Build history of the part. All positions in model axes, mm. A direction names the side the tool comes from. Round coordinates to 2 decimals unless told otherwise and drop trailing zeros. Loops run counter-clockwise (first coordinate to the right, second up) from the corner with the lowest first, then second, coordinate; pieces in that order, holes last. Notation, with made-up numbers: (-40, -26.75) -> (-1, -26.75) arc R33 cw to (-1, 1.25) -> close; hole circle Ø7 at (5, 59). An arc over 180 degrees is marked (long way). Put each result on its own line as item: value. Start each with the question number.
Item 1: Cut at D-D, the plane z = 2. List the corners of the cut face in (x, y), plus the area to 3 significant figures.
Item 2: Drill centre lines: probe 1 along Z at (x, y) = (0.5, 2.2); probe 2 along X at (y, z) = (1.9, 4); probe 3 along X at (y, z) = (4.65, 0.25). Where is each one in solid material? Low to high. Write a range as [from, to].
Item 3: Cut at C-C, the plane y = 0.9. List the corners of the cut face in (x, z).
Item 4: Flat gauge pins, fed straight in: pin 1 Ø2 at (x, y) = (1, 2) entering from -Z; pin 2 Ø3 at (x, z) = (0, 4) entering from -Y. Where does each tip first touch, or does it go through?
Item 5: Cut at B-B, the plane z = 5.25. List the corners of the cut face in (x, y), plus the area to 3 significant figures.
Item 6: Cut at A-A, the plane x = 0. List the corners of the cut face in (y, z), plus the area to 3 significant figures.
Item 7: Pull direction X, two halves, no side cores. Call faces 3 (the cylindrical face through (1.05, 0.74, -8.11)), 4 (the flat face through (-7.8, 1.5, -4.4)), 5 (the cylindrical face through (-0.97, 3.04, -5.27)): +X half, -X half, draft (parallel to the pull), parting line (faces both ways), or undercut.
Item 8: Tool access for faces 1 (the cylindrical face through (-1.17, 3.718, -7.493)), 2 (the cylindrical face through (-0.61, 3.04, 5.48)): list every direction of +Z, -Z, +X, -X, +Y, -Y with a clear straight run to the whole face (end or side of a thin tool).
```python
from build123d import *

# Parameters (mm, degrees)
SKETCH1_R           = 7.5
BOSS_EXTRUDE1_DEPTH = 6
SKETCH2_R           = 8.5
BOSS_EXTRUDE2_DEPTH = 1.5
SKETCH4_R           = 1.6
CUT_EXTRUDE1_DEPTH  = 15.43086969


with BuildPart() as part:
    # Sketch1 → Boss-Extrude1 (new body)
    with BuildSketch(Plane(origin=(0, 0, 0), x_dir=(1, 0, 0), z_dir=(0, 1, 0))):
        with Locations(Location((-1.5, 0, 0), (0, 0, 270))):
            Circle(SKETCH1_R)
    extrude(amount=BOSS_EXTRUDE1_DEPTH)

    # Sketch2 → Boss-Extrude2 (add)
    with BuildSketch(Plane.XZ):
        with Locations(Location((-1.5, 0, 0), (0, 0, 270))):
            Circle(SKETCH2_R)
    extrude(amount=-BOSS_EXTRUDE2_DEPTH)

    # Sketch4 → Cut-Extrude1 (cut, through all)
    with BuildSketch(Plane(origin=(0, 6, 0), x_dir=(1, 0, 0), z_dir=(0, 1, 0))):
        with Locations(Location((0, 4, 0), (0, 0, 270))):
            Circle(SKETCH4_R)
        with Locations(Location((0, -4, 0), (0, 0, 270))):
            Circle(SKETCH4_R)
    extrude(amount=-CUT_EXTRUDE1_DEPTH, mode=Mode.SUBTRACT)


solid = part.part
```
Reply:
1. outline: (-9.76, 0) -> (6.76, 0) -> (6.76, 1.5) -> (5.73, 1.5) -> (5.73, 6) -> (-8.73, 6) -> (-8.73, 1.5) -> (-9.76, 1.5) -> close
1. area: 89.8 mm^2
2. probe 1: z = [-7.23, -5.52], [-2.48, 2.48], [5.52, 7.23]
2. probe 2: x = [-7.84, -1.6], [1.6, 4.84]
2. probe 3: x = [-9, 6]
3. outline: circle Ø17 at (-1.5, 0); hole circle Ø3.2 at (0, -4); hole circle Ø3.2 at (0, 4)
4. pin 1: stops at z = -8.34
4. pin 2: passes through
5. outline: (-8.18, 0) -> (-1, 0) -> (-1, 6) -> (-6.86, 6) -> (-6.86, 1.5) -> (-8.18, 1.5) -> close; (1, 0) -> (5.18, 0) -> (5.18, 1.5) -> (3.86, 1.5) -> (3.86, 6) -> (1, 6) -> close
5. area: 56.3 mm^2
6. outline: (0, -8.37) -> (1.5, -8.37) -> (1.5, -7.35) -> (6, -7.35) -> (6, -5.6) -> (0, -5.6) -> close; (0, -2.4) -> (6, -2.4) -> (6, 2.4) -> (0, 2.4) -> close; (0, 5.6) -> (6, 5.6) -> (6, 7.35) -> (1.5, 7.35) -> (1.5, 8.37) -> (0, 8.37) -> close
6. area: 52.8 mm^2
7. face 3: parting line
7. face 4: draft
7. face 5: undercut
8. face 1: +Y
8. face 2: +Y, -Y
